```python
from build123d import *

# Parameters (mm, degrees)
CROQUIS1_W              = 40
CROQUIS1_H              = 50
SALIENTE_EXTRUIR1_DEPTH = 20
CROQUIS2_R              = 12.5
CORTAR_EXTRUIR1_DEPTH   = 51
CROQUIS3_R              = 1.75
CORTAR_EXTRUIR2_DEPTH   = 21
CORTAR_EXTRUIR3_DEPTH   = 41
CROQUIS5_W              = 5
CROQUIS5_H              = 3
CORTAR_EXTRUIR4_DEPTH   = 3


with BuildPart() as part:
    # Croquis1 → Saliente-Extruir1 (new body)
    with BuildSketch(Plane(origin=(0, 0, 0), x_dir=(1, 0, 0), z_dir=(0, 1, 0))):
        with Locations((20, 25)):
            Rectangle(CROQUIS1_W, CROQUIS1_H)
    extrude(amount=SALIENTE_EXTRUIR1_DEPTH)

    # Croquis2 → Cortar-Extruir1 (cut, through all)
    with BuildSketch(Plane.XY):
        with Locations((20, 20)):
            Circle(CROQUIS2_R)
    extrude(amount=-CORTAR_EXTRUIR1_DEPTH, mode=Mode.SUBTRACT)

    # Croquis3 → Cortar-Extruir2 (cut, through all)
    with BuildSketch(Plane(origin=(0, 20, 0), x_dir=(1, 0, 0), z_dir=(0, 1, 0))):
        with Locations((3.75, 45)):
            Circle(CROQUIS3_R)
        with Locations((36.25, 45)):
            Circle(CROQUIS3_R)
        with Locations((36.25, 5)):
            Circle(CROQUIS3_R)
        with Locations((3.75, 5)):
            Circle(CROQUIS3_R)
    extrude(amount=-CORTAR_EXTRUIR2_DEPTH, mode=Mode.SUBTRACT)

    # Croquis4 → Cortar-Extruir3 (cut, through all)
    with BuildSketch(Plane(origin=(40, 0, 0), x_dir=(0, 0, -1), z_dir=(1, 0, 0))):
        Polygon((25, 20), (37, 20), (37, 8), (13, 8), (13, 20), align=None)
    extrude(amount=-CORTAR_EXTRUIR3_DEPTH, mode=Mode.SUBTRACT)

    # Croquis5 → Cortar-Extruir4 (cut)
    with BuildSketch(Plane(origin=(0, 20, 0), x_dir=(1, 0, 0), z_dir=(0, 1, 0))):
        with Locations((6.25, 38.5)):
            Rectangle(CROQUIS5_W, CROQUIS5_H)
        with Locations((33.75, 38.5)):
            Rectangle(CROQUIS5_W, CROQUIS5_H)
        with Locations((33.75, 11.5)):
            Rectangle(CROQUIS5_W, CROQUIS5_H)
        with Locations((6.25, 11.5)):
            Rectangle(CROQUIS5_W, CROQUIS5_H)
    extrude(amount=-CORTAR_EXTRUIR4_DEPTH, mode=Mode.SUBTRACT)


solid = part.part
```
Input: part model. Units: mm. Frame: model coordinates. A direction names the side the tool comes from. Round coordinates to 2 decimals unless told otherwise and drop trailing zeros. Loops run counter-clockwise (first coordinate to the right, second up) from the corner with the lowest first, then second, coordinate; pieces in that order, holes last. Notation, with made-up numbers: (75.25, -22.75) -> (79.25, -22.75) arc R3 ccw to (79.25, -17.75) -> close; hole circle Ø3 at (13, 79). An arc over 180 degrees is marked (long way). One line per item, written item: value.
(1) Set-up query: faces 1 (the face through (8, 8, -25)), 2 (the face through (3.75, 19, -11)), 3 (the face through (37.06, 10.14, -3.45)). Return all of +Z, -Z, +X, -X, +Y, -Y with unobstructed straight access to the full face (end or side cutting, diameter ignored); none if empty.
Geometry check:
face 1: +X, -X, +Y
face 2: +Y
face 3: +Y, -Y
(2) Pin query (flat end, axial travel): pin 1 (1.5 mm diameter, centred on x = 5.5, z = -11, fed in from +Y); pin 2 (10 mm diameter, centred on x = 26.5, y = 3, fed in from +Z); pin 3 (1 mm diameter, centred on y = 9.5, z = -26.5, fed in from -X); pin 4 (1 mm diameter, centred on x = 5, z = -17.5, fed in from +Y). Return the tip coordinate at first contact, or that it passes through.
Geometry check:
pin 1: y = 17
pin 2: z = 0
pin 3: through
pin 4: y = 8
(3) Material intervals for line 1 (Z direction, x = 36.25, y = 7.25); line 2 (Z direction, x = 36.25, y = 14.75); line 3 (X direction, y = 9.75, z = -5), sorted ascending. Write a range as [from, to].
Geometry check:
line 1: [-50, -46.75], [-43.25, -6.75], [-3.25, 0]
line 2: [-50, -46.75], [-43.25, -37], [-13, -6.75], [-3.25, 0]
line 3: [0, 2], [5.5, 12.85], [27.15, 34.5], [38, 40]
(4) Section B-B (y = 9.25). Return the cut outline in (x, z).
Geometry check:
outline: (0, -50) -> (13.62, -50) -> (13.62, -37) -> (0, -37) -> close; (0, -13) -> (13.62, -13) -> (13.62, 0) -> (0, 0) -> close; (26.38, -50) -> (40, -50) -> (40, -37) -> (26.38, -37) -> close; (26.38, -13) -> (40, -13) -> (40, 0) -> (26.38, 0) -> close; hole circle Ø3.5 at (3.75, -45); hole circle Ø3.5 at (3.75, -5); hole circle Ø3.5 at (36.25, -45); hole circle Ø3.5 at (36.25, -5)
(5) Mould query, pull axis X, two halves, no side actions, for faces 4 (the face through (2, 20, -44)), 5 (the face through (35.87, 10.14, -43.29)), 6 (the face through (0, 7.6, -24.7)). Classes: pulls with the +X half, pulls with the -X half, needs draft (parallel to the pull), parting line crosses it, or undercut.
Geometry check:
face 4: needs draft
face 5: undercut
face 6: pulls with the -X half
(6) Section C-C (z = -41). Return the cut outline in (x, y), plus the area to 3 significant figures.
Geometry check:
outline: (0, 0) -> (40, 0) -> (40, 20) -> (32.5, 20) arc R12.5 cw to (7.5, 20) -> (0, 20) -> close
area: 555 mm2
(7) Section D-D (x = 10.5). Return the cut outline in (y, z), plus the area to 3 significant figures.
Geometry check:
outline: (0, -50) -> (11.88, -50) -> (11.88, -37) -> (8, -37) -> (8, -13) -> (11.88, -13) -> (11.88, 0) -> (0, 0) -> close
area: 501 mm2
(8) Section A-A (y = 6.5). Return the cut outline in (x, z), plus the area to 3 significant figures.
Geometry check:
outline: (0, -50) -> (40, -50) -> (40, 0) -> (0, 0) -> close; hole circle Ø3.5 at (3.75, -45); hole circle Ø3.5 at (3.75, -5); hole circle Ø3.5 at (36.25, -45); hole circle Ø3.5 at (36.25, -5)
area: 1,960 mm2
